The listing builds one solid part. Answer for the finished solid, in the listing's coordinates (mm). Face numbers are marked on the shaded views. Round coordinates to 2 decimals unless told otherwise and drop trailing zeros. Loops run counter-clockwise (first coordinate to the right, second up) from the corner with the lowest first, then second, coordinate; pieces in that order, holes last. Notation, with made-up numbers: M -1.75,47 L 45.25,47 A14 ccw 45.25,70 Z; hole C -8,85.5 d7. An arc over 180 degrees is marked long. Put each result on its own line as item: value. Start each with the question number.
(1) Straight lines are drawn through the part: line 1 (X direction, y = 20, z = -5.5); line 2 (Z direction, x = 14.5, y = 22); line 3 (Z direction, x = -5, y = -20.5). For each, find the intervals that lie inside material, in ascending order.
(2) Section D-D, the plane x = 6 is taken. Determine the outline of the cut face in (y, z).
(3) Section B-B, the plane y = 11 is taken. Determine the outline of the cut face in (x, z), then the cut area to 3 significant figures.
(4) Flat-ended cylindrical pins translate along their axes: P1, Ø6, axis at y = -23, z = -16.5, coming from the +X side; P2, Ø3, axis at x = -0.5, z = -15, coming from the +Y side; P3, Ø4, axis at x = -11.5, y = 19, coming from the -Z side. Find the tip coordinate at first contact, or state that the pin passes through.
(5) Determine the mould class of the marked faces 1, 2, 3 and 4 for opening direction Y: released by +Y, released by -Y, zero draft, split by the parting line, or undercut.
(6) Section C-C, the plane y = -22 is taken. Determine the outline of the cut face in (x, z).
(7) Section A-A, the plane x = 0 is taken. Determine the outline of the cut face in (y, z), then the cut area to 3 significant figures.
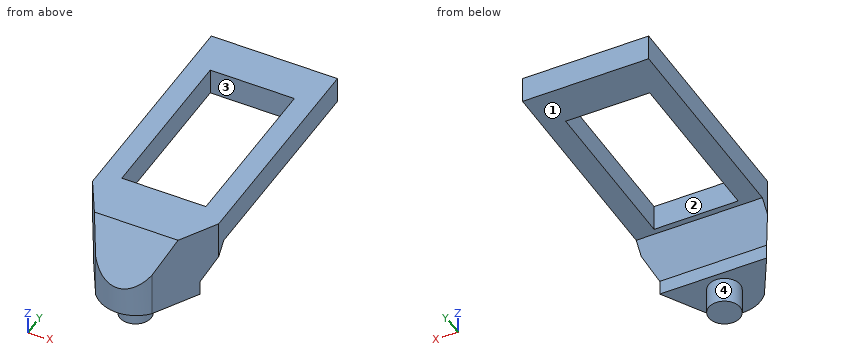
```python
from build123d import *

# Parameters (mm, degrees)
F0_W     = 30.48
F0_H     = 54.61
F0_W_2   = 20.32
F0_H_2   = 40.64
F2_DEPTH = 17.526
F4_START = -25.4
F4_DEPTH = 40.641
F5_R     = 3.81
F6_DEPTH = 6.35


with BuildPart() as f2:
    # F0 (on Top) → F2 (new body)
    with BuildSketch(Plane.XY):
        with Locations((0, 13.335)):
            Rectangle(F0_W, F0_H)
        with Locations((0, 10.16)):
            Rectangle(F0_W_2, F0_H_2, mode=Mode.SUBTRACT)
        with BuildLine():
            Line((15.24, -13.97), (-15.24, -13.97))
            Line((-15.24, -13.97), (-6.8038069676, -28.5819149546))
            ThreePointArc((-6.8038069676, -28.5819149546), (0, -31.75), (6.8038069676, -28.5819149546))
            Line((6.8038069676, -28.5819149546), (15.24, -13.97))
        make_face()
    extrude(amount=-F2_DEPTH)

    # F3 (on Right) → F4 (intersect)
    with BuildSketch(Plane.YZ.offset(F4_START)):
        Polygon((40.7838374376, 0), (0, 0), (-22.86, 0), (-31.9106747376, -10.7861741339), (-31.9106747376, -17.527366057), (-18.003549273, -17.527366057), (-18.003549273, -13.97), (-11.6096100835, -6.35), (40.7838374376, -6.35), align=None)
    extrude(amount=F4_DEPTH, mode=Mode.INTERSECT)

    # F5 (on face) → F6 (join)
    with BuildSketch(Plane(origin=(0, 0, -17.526), x_dir=(1, 0, 0), z_dir=(0, 0, -1))):
        with Locations((0, 23.183679186)):
            Circle(F5_R)
    extrude(amount=F6_DEPTH)


solid = f2.part
```
Recorded:
1. line 1: x = -15.24 to -10.16, 10.16 to 15.24
1. line 2: z = -6.35 to 0
1. line 3: z = -17.53 to 0
2. outline: M -29.42,-17.53 L -18,-17.53 L -18,-13.97 L -11.61,-6.35 L -10.16,-6.35 L -10.16,0 L -22.86,0 L -29.42,-7.82 Z; M 30.48,-6.35 L 40.64,-6.35 L 40.64,0 L 30.48,0 Z
3. outline: M -15.24,-6.35 L -10.16,-6.35 L -10.16,0 L -15.24,0 Z; M 10.16,-6.35 L 15.24,-6.35 L 15.24,0 L 10.16,0 Z
3. area: 64.5 mm²
4. P1: stops at x = 11.76
4. P2: stops at y = -17.61
4. P3: stops at z = -6.35
5. face 1: zero draft
5. face 2: undercut
5. face 3: undercut
5. face 4: split by the parting line
6. outline: M -10.6,-17.53 L -3.62,-17.53 L -3.62,-23.88 L 3.62,-23.88 L 3.62,-17.53 L 10.6,-17.53 L 10.6,0 L -10.6,0 Z
7. outline: M -31.75,-17.53 L -26.99,-17.53 L -26.99,-23.88 L -19.37,-23.88 L -19.37,-17.53 L -18,-17.53 L -18,-13.97 L -11.61,-6.35 L -10.16,-6.35 L -10.16,0 L -22.86,0 L -31.75,-10.59 Z; M 30.48,-6.35 L 40.64,-6.35 L 40.64,0 L 30.48,0 Z
7. area: 381 mm²
